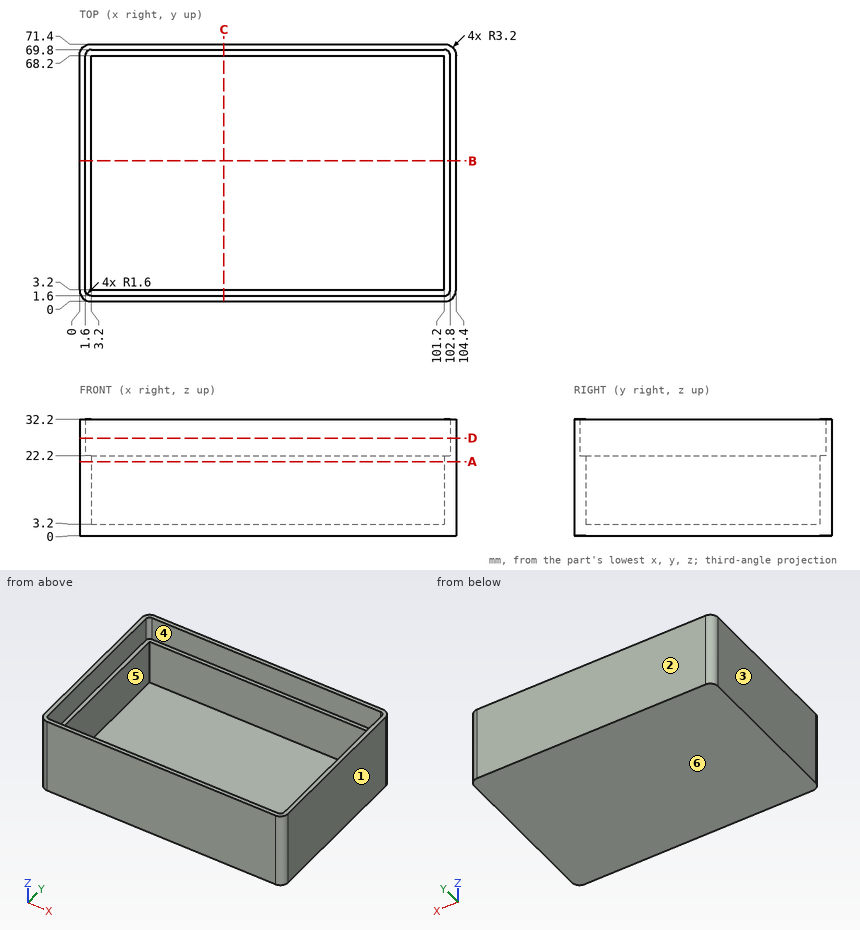
The drawing under review shows one solid part. Ordinate dimensions are in mm from its lowest x, y, z. A direction names the side the tool comes from. Round coordinates to 2 decimals unless told otherwise and drop trailing zeros. Write each loop counter-clockwise with the first axis right and the second up, starting at its lowest first coordinate (ties: lowest second). Pieces come first, ordered by that corner, then holes.
(1) Insertion check: pin 1 (10 mm diameter, centred on x = 18.5, y = 62, fed in from -Z). The pin has a flat end and moves straight along its axis. Give the tip position at first contact, or say it passes through.
(2) Machinability: for the marked faces 5 and 6, which of the approach directions +Z, -Z, +X, -X, +Y, -Y give a long, thin tool a straight path to every point of the face, cutting with its end or side? Answer none if there is none.
(3) We need section C-C on x = 40. Give the boundary of the cut face in (y, z).
(4) We need section B-B on y = 39. Give the boundary of the cut face in (x, z).
(5) We need section A-A on z = 20.5. Give the boundary of the cut face in (x, y), and give its area (3 significant figures).
(6) We need section D-D on z = 27. Give the boundary of the cut face in (x, y), and give its area (3 significant figures).
(7) Wall thickness on L1, parallel to Y at x = 78.5, z = 17.5; L2, parallel to X at y = 49, z = 6; L3, parallel to Y at x = 37, z = 25: over which ranges is each line inside the solid? List them lowest first.
(8) Mouldability with a two-part tool opening along X and no side actions: class the marked faces 1, 2, 3 and 4 as +X half, -X half, draft (parallel to the pull), parting line (faces both ways), or undercut.
Findings below:
1. pin 1: stops at z = 0
2. face 5: +Z
2. face 6: -Z, +X, -X, +Y, -Y
3. outline: (0, 0) - (71.4, 0) - (71.4, 32.2) - (69.8, 32.2) - (69.8, 22.2) - (68.2, 22.2) - (68.2, 3.2) - (3.2, 3.2) - (3.2, 22.2) - (1.6, 22.2) - (1.6, 32.2) - (0, 32.2) - close
4. outline: (0, 0) - (104.4, 0) - (104.4, 32.2) - (102.8, 32.2) - (102.8, 22.2) - (101.2, 22.2) - (101.2, 3.2) - (3.2, 3.2) - (3.2, 22.2) - (1.6, 22.2) - (1.6, 32.2) - (0, 32.2) - close
5. outline: (0, 3.2) arc R3.2 ccw to (3.2, 0) - (101.2, 0) arc R3.2 ccw to (104.4, 3.2) - (104.4, 68.2) arc R3.2 ccw to (101.2, 71.4) - (3.2, 71.4) arc R3.2 ccw to (0, 68.2) - close; hole (3.2, 3.2) - (101.2, 3.2) - (101.2, 68.2) - (3.2, 68.2) - close
5. area: 1,080 mm2
6. outline: (0, 3.2) arc R3.2 ccw to (3.2, 0) - (101.2, 0) arc R3.2 ccw to (104.4, 3.2) - (104.4, 68.2) arc R3.2 ccw to (101.2, 71.4) - (3.2, 71.4) arc R3.2 ccw to (0, 68.2) - close; hole (1.6, 3.2) arc R1.6 ccw to (3.2, 1.6) - (101.2, 1.6) arc R1.6 ccw to (102.8, 3.2) - (102.8, 68.2) arc R1.6 ccw to (101.2, 69.8) - (3.2, 69.8) arc R1.6 ccw to (1.6, 68.2) - close
6. area: 546 mm2
7. L1: y = 0 to 3.2, 68.2 to 71.4
7. L2: x = 0 to 3.2, 101.2 to 104.4
7. L3: y = 0 to 1.6, 69.8 to 71.4
8. face 1: +X half
8. face 2: draft
8. face 3: -X half
8. face 4: undercut
